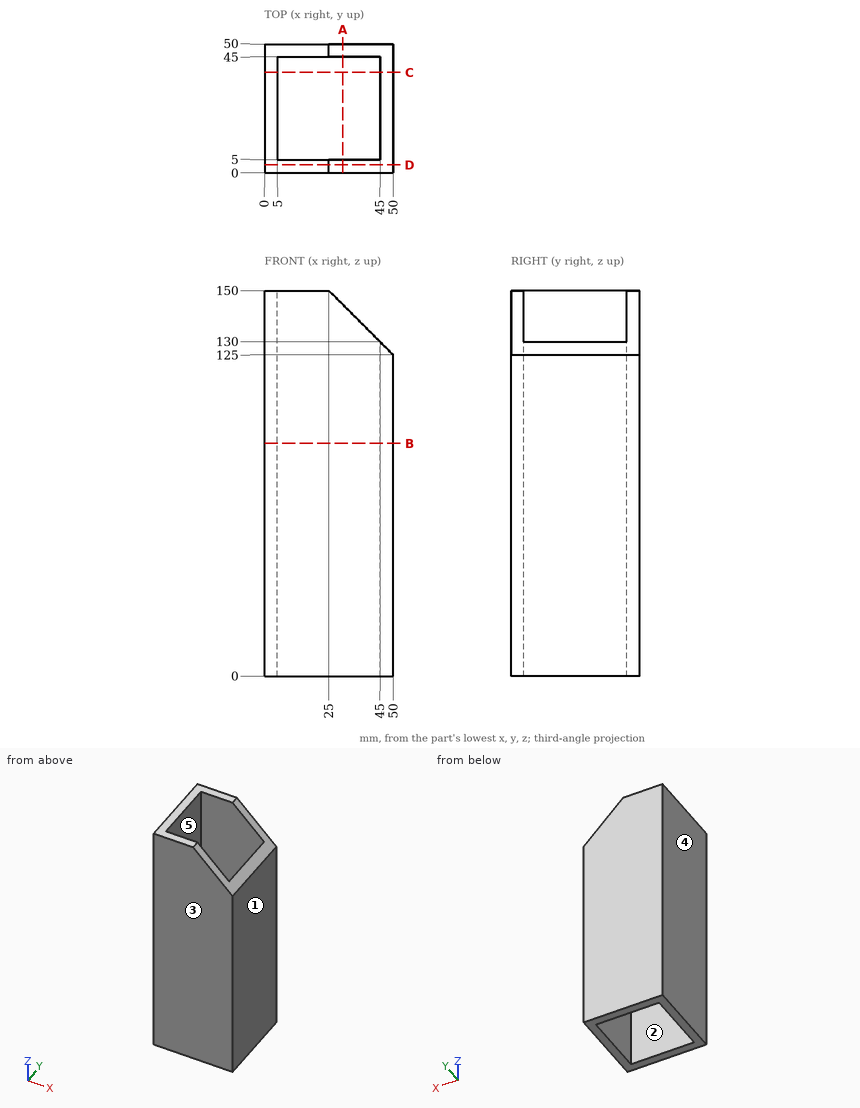
Input: dimensioned drawing with shaded views. Units: mm. Origin: part minimum x, y, z. A direction names the side the tool comes from. Give positions to 0.01 mm unless a question says otherwise; leave off trailing zeros. Write each loop counter-clockwise with the first axis right and the second up, starting at its lowest first coordinate (ties: lowest second). Pieces come first, ordered by that corner, then holes. Notation, with made-up numbers: (71.25, 49.5) -> (78.25, 49.5) arc R30 ccw to (78.25, 81.5) -> close; hole circle Ø8 at (-34, 14). An arc over 180 degrees is marked (long way). Answer as a JSON object with one key per item and string values.
1. Cut plane C-C on y = 39. Output: boundary loops of the cut face in (x, z).
Ans:
{"outline": "(0, 0) -> (5, 0) -> (5, 150) -> (0, 150) -> close; (45, 0) -> (50, 0) -> (50, 125) -> (45, 130) -> close"}
2. Ray query, probe 1 along Y at (x, z) = (27.5, 53); probe 2 along X at (y, z) = (37.5, 133). Return the intervals inside material, ascending. Write a range as from..to.
Ans:
{"probe 1": "y = 0..5, 45..50", "probe 2": "x = 0..5"}
3. Mould query, pull axis X, two halves, no side actions, for the marked faces 3, 4 and 5. Classes: pulls with the +X half, pulls with the -X half, needs draft (parallel to the pull), parting line crosses it, or undercut.
Ans:
{"face 3": "needs draft", "face 4": "pulls with the -X half", "face 5": "undercut"}
4. Access query for the marked faces 1 and 2. Directions: +Z, -Z, +X, -X, +Y, -Y. A direction counts if a zero-diameter tool reaches every point of the face in a straight line with its end or side. Return the directions, or none.
Ans:
{"face 1": "+Z, -Z, +X, +Y, -Y", "face 2": "+Z, -Z"}
5. Cut plane D-D on y = 3. Output: boundary loops of the cut face in (x, z).
Ans:
{"outline": "(0, 0) -> (50, 0) -> (50, 125) -> (25, 150) -> (0, 150) -> close"}
6. Contact query for flat-ended pins moving along their axis: pin 1 (1.5 mm diameter, centred on x = 16.5, y = 6.5, fed in from +Z); pin 2 (10 mm diameter, centred on x = 45, y = 19.5, fed in from -Z). Output: stop coordinate, or through.
Ans:
{"pin 1": "passes through", "pin 2": "stops at z = 0"}
7. Cut plane B-B on z = 90.5. Output: boundary loops of the cut face in (x, y).
Ans:
{"outline": "(0, 0) -> (50, 0) -> (50, 50) -> (0, 50) -> close; hole (5, 5) -> (45, 5) -> (45, 45) -> (5, 45) -> close"}
8. Cut plane A-A on x = 30.5. Output: boundary loops of the cut face in (y, z), and give its area (4 significant figures).
Ans:
{"outline": "(0, 0) -> (5, 0) -> (5, 144.5) -> (0, 144.5) -> close; (45, 0) -> (50, 0) -> (50, 144.5) -> (45, 144.5) -> close", "area": "1,445 mm^2"}
